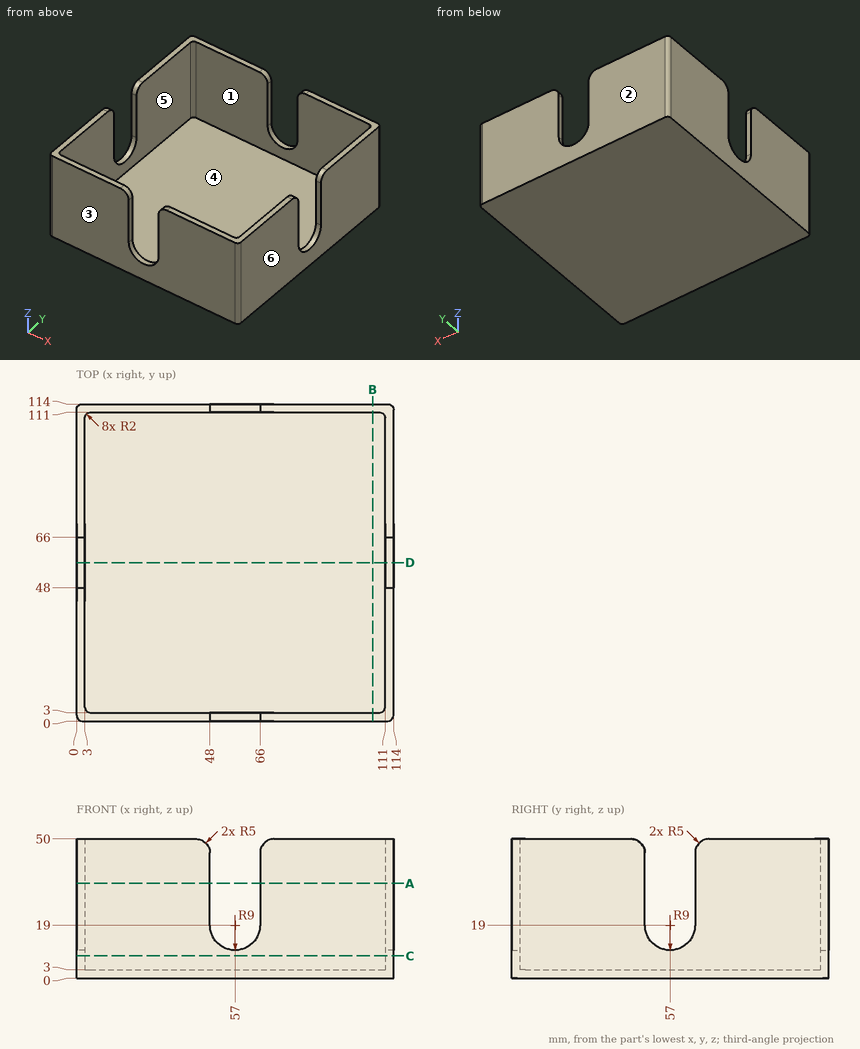
The figure shows three views and two pictorial views of one solid part (mm, origin at its lowest corner). Answer the questions. A direction names the side the tool comes from. Give positions to 0.01 mm unless a question says otherwise; leave off trailing zeros. Write each loop counter-clockwise with the first axis right and the second up, starting at its lowest first coordinate (ties: lowest second). Pieces come first, ordered by that corner, then holes. Notation, with made-up numbers: (50, 56.25) -> (103, 56.25) arc R19 cw to (103, 63.25) -> close; hole circle Ø9 at (75, 10.5). An arc over 180 degrees is marked (long way). Answer as a JSON object with one key per item and string values.
1) Section D-D on y = 57 is taken. Write down the section's boundary in (x, z), then the cut area to 3 significant figures.
Findings below:
{"outline": "(0, 0) -> (114, 0) -> (114, 10) -> (111, 10) -> (111, 3) -> (3, 3) -> (3, 10) -> (0, 10) -> close", "area": "384 mm^2"}
2) A tool of negligible diameter and unlimited length cuts with its end or side. For the marked faces 1 and 2, from which of +Z, -Z, +X, -X, +Y, -Y can it reach the whole face along a straight path? Write none if from no direction.
Findings below:
{"face 1": "+Z", "face 2": "+Z, -Z, +X, -X, +Y"}
3) Straight lines are drawn through the part: probe 1 along Y at (x, z) = (44, 17); probe 2 along Z at (x, y) = (20.5, 87). For each, find the intervals that lie inside material, in ascending order. Write a range as from..to.
Findings below:
{"probe 1": "y = 0..3, 111..114", "probe 2": "z = 0..3"}
4) Section B-B on x = 106.5 is taken. Write down the section's boundary in (y, z).
Findings below:
{"outline": "(0, 0) -> (114, 0) -> (114, 50) -> (111, 50) -> (111, 3) -> (3, 3) -> (3, 50) -> (0, 50) -> close"}
5) Section A-A on z = 34 is taken. Count the separate pieces of the cut face and the enclosed holes in it, then the cut area to 3 significant figures.
Findings below:
{"separate pieces": "4", "enclosed holes": "0", "area": "1,120 mm^2"}
6) Section C-C on z = 8 is taken. Write down the section's boundary in (x, y), then the cut area to 3 significant figures.
Findings below:
{"outline": "(0, 2) arc R2 ccw to (2, 0) -> (112, 0) arc R2 ccw to (114, 2) -> (114, 112) arc R2 ccw to (112, 114) -> (2, 114) arc R2 ccw to (0, 112) -> close; hole (3, 5) arc R2 ccw to (5, 3) -> (109, 3) arc R2 ccw to (111, 5) -> (111, 109) arc R2 ccw to (109, 111) -> (5, 111) arc R2 ccw to (3, 109) -> close", "area": "1,330 mm^2"}
7) Flat-ended cylindrical pins translate along their axes: pin 1 Ø1.5 at (x, z) = (1, 38.5) entering from -Y; pin 2 Ø5 at (x, y) = (58, 92) entering from +Z; pin 3 Ø1.5 at (x, z) = (1, 36.5) entering from +Y. Find the tip coordinate at first contact, or state that the pin passes through.
Findings below:
{"pin 1": "stops at y = 0.02", "pin 2": "stops at z = 3", "pin 3": "stops at y = 113.98"}
8) For a pull along Y with two mould halves and no side action, classify the marked faces 3, 4, 5 and 6 as pulls with the +Y half, pulls with the -Y half, needs draft (parallel to the pull), parting line crosses it, or undercut.
Findings below:
{"face 3": "pulls with the -Y half", "face 4": "undercut", "face 5": "undercut", "face 6": "needs draft"}
